Verification items for the finished model (mm, model axes). Round coordinates to 2 decimals unless told otherwise and drop trailing zeros. Order: outer loops, then holes, each group sorted by start corner. A loop starts at its lowest first (then second) coordinate and runs counter-clockwise, first axis right, second up. Notation, with made-up numbers: M 41.25,89.5 L 52.25,89.5 A17 cw 52.25,98.5 Z; hole C 78.5,59 d3. An arc over 180 degrees is marked long. Use one line per item in the form item = value. Start each with the question number.
Item 1: Cross-section at A-A on z = -49.53. Enter the section's corners in (x, y), then the cut area to 3 significant figures.
Item 2: Thickness scan on probe 1 along X at (y, z) = (0.55, -49.53); probe 2 along Z at (x, y) = (84, 0.9); probe 3 along Z at (x, y) = (109, 0.95). Record the ranges inside material, lowest first. Write a range as [from, to].
Item 3: Cross-section at B-B on x = 57.15. Enter the section's corners in (y, z), then the cut area to 3 significant figures.
Item 4: Release check for a two-part mould opening along X. For faces 1 (the cylindrical face through (118.74, 0.8, 61.69)), 2 (the cylindrical face through (84.263, 0.783, 50.622)), 3 (the flat face through (76, 0, -1)), 4 (the cylindrical face through (34, 1, -62)) record: +X half, -X half, draft (parallel to the pull), parting line (faces both ways), or undercut.
from build123d import *

# Parameters (mm, degrees)
SKETCH1_W           = 241.3
SKETCH1_H           = 127
SKETCH1_R           = 2.032
BOSS_EXTRUDE1_DEPTH = 1.5875
SKETCH2_W           = 152.4
SKETCH2_H           = 127
CUT_EXTRUDE1_DEPTH  = 137.349523858
FILLET2_R           = 6.35


with BuildPart() as part:
    # Sketch1 → Boss-Extrude1 (new body)
    with BuildSketch(Plane(origin=(0, 0, 0), x_dir=(1, 0, 0), z_dir=(0, 1, 0))):
        Rectangle(SKETCH1_W, SKETCH1_H)
        with Locations(Location((82.55, 49.53, 0), (0, 0, 270))):
            Circle(SKETCH1_R, mode=Mode.SUBTRACT)
        with Locations(Location((82.55, -49.53, 0), (0, 0, 270))):
            Circle(SKETCH1_R, mode=Mode.SUBTRACT)
        with Locations(Location((107.95, -49.53, 0), (0, 0, 270))):
            Circle(SKETCH1_R, mode=Mode.SUBTRACT)
        with Locations(Location((107.95, 49.53, 0), (0, 0, 270))):
            Circle(SKETCH1_R, mode=Mode.SUBTRACT)
        with Locations(Location((57.15, -35.4965, 0), (0, 0, 270))):
            Circle(SKETCH1_R, mode=Mode.SUBTRACT)
        with Locations(Location((44.45, -35.4965, 0), (0, 0, 270))):
            Circle(SKETCH1_R, mode=Mode.SUBTRACT)
        with Locations(Location((44.45, -48.1965, 0), (0, 0, 270))):
            Circle(SKETCH1_R, mode=Mode.SUBTRACT)
        with Locations(Location((57.15, -48.1965, 0), (0, 0, 270))):
            Circle(SKETCH1_R, mode=Mode.SUBTRACT)
    extrude(amount=BOSS_EXTRUDE1_DEPTH)

    # Sketch2 → Cut-Extrude1 (cut, through all)
    with BuildSketch(Plane(origin=(0, 1.5875, 0), x_dir=(1, 0, 0), z_dir=(0, 1, 0))):
        with Locations((-44.45, 0)):
            Rectangle(SKETCH2_W, SKETCH2_H)
    extrude(amount=-CUT_EXTRUDE1_DEPTH, mode=Mode.SUBTRACT)

    # Fillet2
    fillet2_edges = [part.edges().sort_by_distance(p)[0] for p in [
        (120.65, 0.79375, 63.5),
        (120.65, 0.79375, -63.5),
        (31.75, 0.79375, -63.5),
        (31.75, 0.79375, 63.5),
    ]]
    fillet(fillet2_edges, radius=FILLET2_R)


solid = part.part
Output values:
q1.outline = M 31.75,0 L 80.52,0 L 80.52,1.59 L 31.75,1.59 Z; M 84.58,0 L 105.92,0 L 105.92,1.59 L 84.58,1.59 Z; M 109.98,0 L 120.65,0 L 120.65,1.59 L 109.98,1.59 Z
q1.area = 128 mm2
q2.probe_1 = [31.75, 80.52], [84.58, 105.92], [109.98, 120.65]
q2.probe_2 = [-63.5, -50.95], [-48.11, 48.11], [50.95, 63.5]
q2.probe_3 = [-63.5, -51.27], [-47.79, 47.79], [51.27, 63.5]
q3.outline = M 0,-63.5 L 1.59,-63.5 L 1.59,33.46 L 0,33.46 Z; M 0,37.53 L 1.59,37.53 L 1.59,46.16 L 0,46.16 Z; M 0,50.23 L 1.59,50.23 L 1.59,63.5 L 0,63.5 Z
q3.area = 189 mm2
q4.face_1 = +X half
q4.face_2 = undercut
q4.face_3 = draft
q4.face_4 = -X half
